Job drawing, mm, ordinate dimensions from the low corner. One solid piece. A direction names the side the tool comes from. Round coordinates to 2 decimals unless told otherwise and drop trailing zeros. Loops run counter-clockwise (first coordinate to the right, second up) from the corner with the lowest first, then second, coordinate; pieces in that order, holes last.
1) 3-axis set-ups, long thin cutter, end or side, ignore diameter. For the marked faces 1 and 2: which of +Z, -Z, +X, -X, +Y, -Y reach the whole face in a straight line?
2) Band-saw the part on D-D, the plane y = 21.75. Write the cut outline in (x, z).
3) Drop flat-ended pins along their axis: P1, Ø8, axis at x = 15, z = 10, coming from the +Y side; P2, Ø1.5, axis at x = 25.5, z = 4, coming from the +Y side. Give the stop position or say it passes through.
4) Probe line 1 (X direction, y = 15.25, z = 11); line 2 (Y direction, x = 0.75, z = 15); line 3 (X direction, y = 1.1, z = 10). List the from-to ranges inside material, lowest first.
5) Band-saw the part on B-B, the plane y = 11. Write the cut outline in (x, z).
6) Band-saw the part on C-C, the plane z = 13.5. Write the cut outline in (x, y).
7) Band-saw the part on A-A, the plane x = 15. Write the cut outline in (y, z).
8) Mould opens along X. For the marked faces 3, 4 and 5 say: +X half, -X half, draft (parallel to the pull), parting line (faces both ways), or undercut.
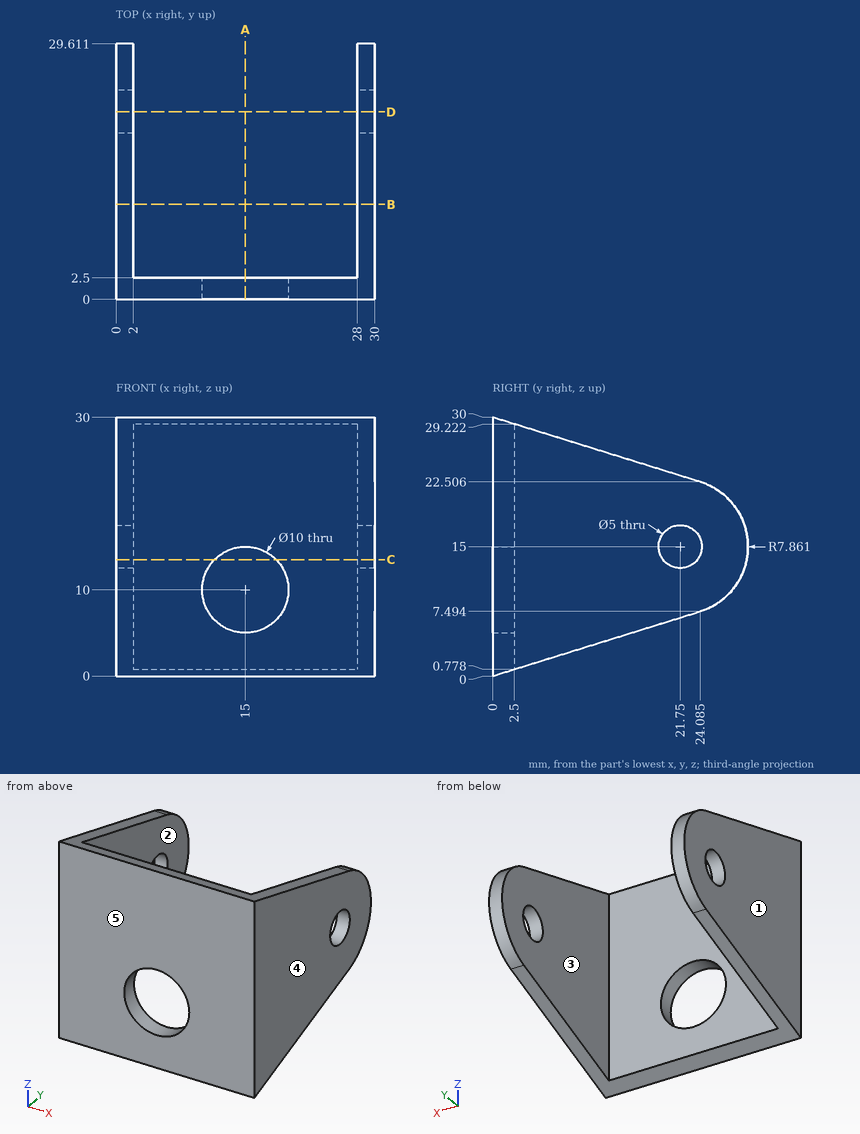
Reported:
1. face 1: +Z, -Z, -X, +Y, -Y
1. face 2: +Z, -Z, +Y
2. outline: (0, 6.77) - (2, 6.77) - (2, 12.5) - (0, 12.5) - close; (0, 17.5) - (2, 17.5) - (2, 23.23) - (0, 23.23) - close; (28, 6.77) - (30, 6.77) - (30, 12.5) - (28, 12.5) - close; (28, 17.5) - (30, 17.5) - (30, 23.23) - (28, 23.23) - close
3. P1: passes through
3. P2: stops at y = 2.5
4. line 1: x = 0 to 2, 28 to 30
4. line 2: y = 0 to 19.25, 24.25 to 29.61
4. line 3: x = 0 to 10, 20 to 30
5. outline: (0, 3.42) - (2, 3.42) - (2, 26.58) - (0, 26.58) - close; (28, 3.42) - (30, 3.42) - (30, 26.58) - (28, 26.58) - close
6. outline: (0, 0) - (11.43, 0) - (11.43, 2.5) - (2, 2.5) - (2, 19.75) - (0, 19.75) - close; (0, 23.75) - (2, 23.75) - (2, 29.47) - (0, 29.47) - close; (18.57, 0) - (30, 0) - (30, 19.75) - (28, 19.75) - (28, 2.5) - (18.57, 2.5) - close; (28, 23.75) - (30, 23.75) - (30, 29.47) - (28, 29.47) - close
7. outline: (0, 0) - (2.5, 0.78) - (2.5, 5) - (0, 5) - close; (0, 15) - (2.5, 15) - (2.5, 29.22) - (0, 30) - close
8. face 3: undercut
8. face 4: +X half
8. face 5: draft
